from build123d import *

# Parameters (mm, degrees)
F1_DEPTH = 30
F2_R     = 5
F3_DEPTH = 30
F4_DEPTH = 30


with BuildPart() as f1:
    # F0 (on Front) → F1 (new body)
    with BuildSketch(Plane.XZ):
        Polygon((-50, 100), (-50, 0), (-50, -100), (0, -100), (50, -100), (50, 0), (50, 100), (0, 100), align=None)
    extrude(amount=F1_DEPTH)

    # F2 (on face) → F3 (cut)
    with BuildSketch(Plane.XZ.offset(30)):
        with Locations((0, 60)):
            Circle(F2_R)
    extrude(amount=-F3_DEPTH, mode=Mode.SUBTRACT)

    # F2 (on face) → F4 (cut)
    with BuildSketch(Plane.XZ.offset(30)):
        with Locations((0, -20)):
            Circle(F2_R)
        with Locations((0, 60)):
            Circle(F2_R)
    extrude(amount=-F4_DEPTH, mode=Mode.SUBTRACT)


solid = f1.part
Geometry check sheet. Reference: the model listing, model coordinates, mm. Round coordinates to 2 decimals unless told otherwise and drop trailing zeros. Loops run counter-clockwise (first coordinate to the right, second up) from the corner with the lowest first, then second, coordinate; pieces in that order, holes last. Notation, with made-up numbers: (-34, 76.5) - (12, 76.5) arc R29 cw to (12, 100.5) - close; hole circle Ø8 at (21, 66). An arc over 180 degrees is marked (long way). One line per question, with ' | ' between items. Start each with the question number.
1. Scan lines: line 1 (Z direction, x = 0, y = -15.5); line 2 (Z direction, x = 4.5, y = -6.5); line 3 (X direction, y = -28.5, z = 58). Record each from-to range of solid material in increasing order. Write a range as [from, to].
2. Cross-section at A-A on z = -20. Record the cut outline in (x, y).
3. Draft check along X on faces 1 (the face through (1, -15, 100)), 2 (the face through (50, -15, -1)), 3 (the face through (3, -15, 64)), 4 (the face through (-1.08, -15.21, -24.88)). Enter one of: released by +X, released by -X, zero draft, split by the parting line, or undercut.
4. Cross-section at B-B on x = 0. Record the cut outline in (y, z), then the cut area to 3 significant figures.
Taken from the geometry:
1) line 1: [-100, -25], [-15, 55], [65, 100] | line 2: [-100, -22.18], [-17.82, 57.82], [62.18, 100] | line 3: [-50, -4.58], [4.58, 50]
2) outline: (-50, -30) - (-5, -30) - (-5, 0) - (-50, 0) - close; (5, -30) - (50, -30) - (50, 0) - (5, 0) - close
3) face 1: zero draft | face 2: released by +X | face 3: undercut | face 4: undercut
4) outline: (-30, -100) - (0, -100) - (0, -25) - (-30, -25) - close; (-30, -15) - (0, -15) - (0, 55) - (-30, 55) - close; (-30, 65) - (0, 65) - (0, 100) - (-30, 100) - close | area: 5,400 mm²
